Source: CAD feature listing. Evaluate the final solid. Frame: model axes, mm. A direction names the side the tool comes from. Give positions to 0.01 mm unless a question says otherwise; leave off trailing zeros. Order: outer loops, then holes, each group sorted by start corner. A loop starts at its lowest first (then second) coordinate and runs counter-clockwise, first axis right, second up.
1) Section B-B, the plane x = 21.5. Return loops of the section in (y, z).
2) First-contact query: P1, Ø5, axis at x = -43.5, z = 2, coming from the +Y side; P2, Ø5, axis at y = 19.5, z = 3, coming from the +X side; P3, Ø10, axis at y = -20.5, z = -9.5, coming from the +X side; P4, Ø14.5, axis at x = 0, z = 13.335, coming from the +Y side. Flat tips, straight axial feed; report the tip coordinate or a pass-through.
3) Material intervals for line 1 (X direction, y = 17, z = 13); line 2 (Y direction, x = 28.5, z = -3.5); line 3 (Z direction, x = 0, y = 19) (1 decimal), sorted ascending.
4) Section A-A, the plane y = 0. Return loops of the section in (x, z).
5) Access query for faces 5 (the face through (-10.341, -19, -6)), 6 (the face through (0, 12.7, 3)), 7 (the face through (-14.278, 19, 6)). Directions: +Z, -Z, +X, -X, +Y, -Y. A direction counts if a zero-diameter tool reaches every point of the face in a straight line with its end or side. Return the directions, or none.
6) Draft query along X for faces 1 (the face through (31.96, 25.37, -6.26)), 2 (the face through (21, -12.7, -6)), 3 (the face through (-21, -25.4, -6)), 4 (the face through (-56.144, -0.654, -6.261)). Return one class per face: released by +X, released by -X, zero draft, split by the parting line, or undercut.
```python
from build123d import *

# Parameters (mm, degrees)
F1_DEPTH = 12.7
F2_R     = 6.35
F3_DEPTH = 12.7


with BuildPart() as f1:
    # F0 (on Top) → F1 (new body)
    with BuildSketch(Plane.XY):
        with BuildLine():
            ThreePointArc((30.752141, 12.7), (43.452141, 0), (30.752141, -12.7))
            Line((30.752141, -12.7), (10.341428, -12.7))
            Line((10.341428, -12.7), (10.341428, -25.4))
            Line((10.341428, -25.4), (30.752141, -25.4))
            ThreePointArc((30.752141, -25.4), (56.123977, -1.195799), (33.141087, 25.287407))
            Line((33.141087, 25.287407), (30.752141, 25.295523))
            Line((30.752141, 25.295523), (30.752141, 12.7))
        make_face()
        with BuildLine():
            Line((0, 12.7), (30.752141, 12.7))
            Line((30.752141, 12.7), (30.752141, 25.295523))
            Line((30.752141, 25.295523), (0, 25.4))
            Line((0, 25.4), (-33.141087, 25.287407))
            ThreePointArc((-33.141087, 25.287407), (-56.123977, -1.195799), (-30.752141, -25.4))
            Line((-30.752141, -25.4), (-10.341428, -25.4))
            Line((-10.341428, -25.4), (-10.341428, -12.7))
            Line((-10.341428, -12.7), (-30.752141, -12.7))
            ThreePointArc((-30.752141, -12.7), (-43.452141, 0), (-30.752141, 12.7))
            Line((-30.752141, 12.7), (0, 12.7))
        make_face()
        Polygon((0, 25.4), (30.752141, 25.295523), (30.752141, 25.4), align=None)
        with BuildLine():
            Line((30.752141, 25.4), (30.752141, 25.295523))
            Line((30.752141, 25.295523), (33.141087, 25.287407))
            ThreePointArc((33.141087, 25.287407), (31.94794, 25.371836), (30.752141, 25.4))
        make_face()
    extrude(amount=-F1_DEPTH)

    # F2 (on face) → F3 (join)
    with BuildSketch(Plane.XZ.offset(-12.7)):
        with BuildLine():
            Line((14.2875, 0), (14.2875, 13.335001))
            ThreePointArc((14.2875, 13.335001), (-0.263015, 27.62008), (-14.277816, 12.809059))
            Line((-14.277816, 12.809059), (-14.277816, 0))
            Line((-14.277816, 0), (14.2875, 0))
        make_face()
        with Locations((0, 13.335001)):
            Circle(F2_R, mode=Mode.SUBTRACT)
    extrude(amount=-F3_DEPTH)


solid = f1.part
```
From the geometry:
1. outline: (-25.4, -12.7) - (-12.7, -12.7) - (-12.7, 0) - (-25.4, 0) - close; (12.7, -12.7) - (25.4, -12.7) - (25.4, 0) - (12.7, 0) - close
2. P1: stops at y = 22.77
2. P2: stops at x = 14.29
2. P3: stops at x = 50.87
2. P4: stops at y = 25.4
3. line 1: x = -14.28 to -6.34, 6.34 to 14.29
3. line 2: y = -25.4 to -12.7, 12.7 to 25.4
3. line 3: z = -12.7 to 7, 19.7 to 27.6
4. outline: (-56.15, -12.7) - (-43.45, -12.7) - (-43.45, 0) - (-56.15, 0) - close; (43.45, -12.7) - (56.15, -12.7) - (56.15, 0) - (43.45, 0) - close
5. face 5: +Z, -Z, -Y
5. face 6: +Z, -Z
5. face 7: +Z, -X, +Y, -Y
6. face 1: released by +X
6. face 2: undercut
6. face 3: zero draft
6. face 4: released by -X
